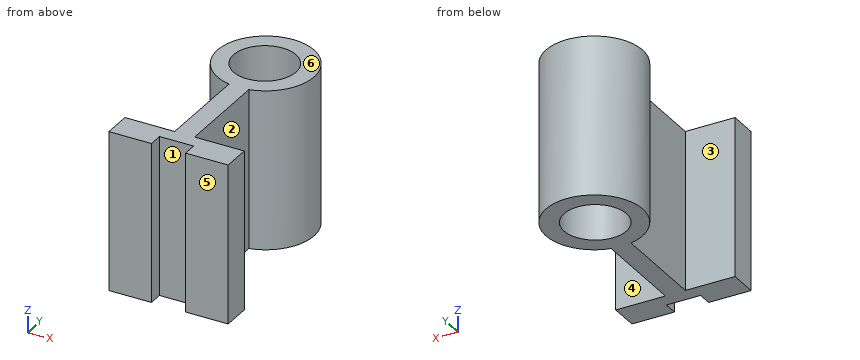
```python
from build123d import *

# Parameters (mm, degrees)
SKETCH3_R           = 11
BOSS_EXTRUDE1_DEPTH = 56


with BuildPart() as part:
    # Sketch3 → Boss-Extrude1 (new body)
    with BuildSketch(Plane.XY):
        with BuildLine():
            Line((0, 0), (-15, 0))
            Line((-15, 0), (-15, 10))
            Line((-15, 10), (2.5, 10))
            Line((2.5, 10), (2.5, 43.750570873))
            ThreePointArc((2.5, 43.750570873), (6, 77.386375632), (9.5, 43.750570873))
            Line((9.5, 43.750570873), (9.5, 10))
            Line((9.5, 10), (27, 10))
            Line((27, 10), (27, 0))
            Line((27, 0), (12, 0))
            Line((12, 0), (12, 5))
            Line((12, 5), (0, 5))
            Line((0, 5), (0, 0))
        make_face()
        with Locations((5.728023625, 60.256681192)):
            Circle(SKETCH3_R, mode=Mode.SUBTRACT)
    extrude(amount=BOSS_EXTRUDE1_DEPTH)


solid = part.part
```
The listing builds one solid part. Answer for the finished solid, in the listing's coordinates (mm). Face numbers are marked on the shaded views. A direction names the side the tool comes from. Give positions to 0.01 mm unless a question says otherwise; leave off trailing zeros. Order: outer loops, then holes, each group sorted by start corner. A loop starts at its lowest first (then second) coordinate and runs counter-clockwise, first axis right, second up. Notation, with made-up numbers: (-8, 73.5) - (1, 73.5) arc R5 cw to (1, 78.5) - close; hole circle Ø6 at (41, 73.25). An arc over 180 degrees is marked (long way). Answer in a Markdown table with one row per item. Add a question column.
Q1. For a pull along Y with two mould halves and no side action, classify the marked faces 4, 5 and 6 as released by +Y, released by -Y, zero draft, split by the parting line, or undercut.
Q2. Which of the six approach directions +Z, -Z, +X, -X, +Y, -Y give full straight-line access (tool end or side, diameter ignored) to the marked faces 1, 2 and 3?
Q3. The part is cut by section C-C (y = 28). Determine the outline of the cut face in (x, z).
Q4. Given P1, Ø5, axis at x = 22, z = 28.5, coming from the +Y side; P2, Ø8, axis at x = 12, z = 8, coming from the +Y side; P3, Ø6, axis at x = -2.5, z = 18, coming from the +Y side, each flat-ended and moving along its own axis, determine where each tip first touches the part or whether it passes through.
Q5. Find the intervals of material crossed by line 1 along Y through (x, z) = (10.5, 21.5); line 2 along Y through (x, z) = (2, 25); line 3 along X through (y, z) = (29, 26.5), in increasing order. Write a range as [from, to].
Q6. The part is cut by section A-A (x = 8). Determine the outline of the cut face in (y, z).
Q7. The part is cut by section B-B (z = 49). Determine the outline of the cut face in (x, y), then the cut area to 3 significant figures.
Determined:
| question | item | result |
|---|---|---|
| 1 | face 4 | undercut |
| 1 | face 5 | released by -Y |
| 1 | face 6 | zero draft |
| 2 | face 1 | +Z, -Z, -Y |
| 2 | face 2 | +Z, -Z, +X |
| 2 | face 3 | +Z, -Z, -X |
| 3 | outline | (2.5, 0) - (9.5, 0) - (9.5, 56) - (2.5, 56) - close |
| 4 | P1 | stops at y = 70.72 |
| 4 | P2 | stops at y = 77.27 |
| 4 | P3 | stops at y = 76.47 |
| 5 | line 1 | y = [5, 10], [43.99, 50.35], [70.17, 76.78] |
| 5 | line 2 | y = [5, 10], [43.86, 49.91], [70.61, 76.91] |
| 5 | line 3 | x = [2.5, 9.5] |
| 6 | outline | (5, 0) - (49.49, 0) - (49.49, 56) - (5, 56) - close; (71.02, 0) - (77.27, 0) - (77.27, 56) - (71.02, 56) - close |
| 7 | outline | (-15, 0) - (0, 0) - (0, 5) - (12, 5) - (12, 0) - (27, 0) - (27, 10) - (9.5, 10) - (9.5, 43.75) arc R17 ccw (long way) to (2.5, 43.75) - (2.5, 10) - (-15, 10) - close; hole circle Ø22 at (5.73, 60.26) |
| 7 | area | 1,120 mm² |
